Autodesk Inventor part; units mm, degrees
ref_plane "YZ Plane" through (0, 0, 0) normal (1, 0, 0) x (0, 1, 0)
ref_plane "XZ Plane" through (0, 0, 0) normal (0, 1, 0) x (-1, 0, 0)
ref_plane "XY Plane" through (0, 0, 0) normal (0, 0, 1) x (1, 0, 0)
sketch "Sketch1" plane through (0, 0, 0) normal (0, 0, 1) x (1, 0, 0)
  arc A0 (187.325, 0) -> (0, 187.325) centre (0, 0) ccw
  arc A1 (136.525, 0) -> (0, 136.525) centre (0, 0) ccw
  line L0 (0, 136.525) -> (0, 187.325)
  line L1 (136.525, 0) -> (187.325, 0)
  point P0 (161.925, 0)
  point P1 (0, 161.925)
  dimension "d2" = 187.325
  dimension "d3" = 136.525
extrude "Extrusion1" add sketch "Sketch1" along normal blind 0.4
sketch "Sketch3" plane through (0, 0, 0.4) normal (0, 0, 1) x (1, 0, 0)
  arc A0 (178.117, 32.1925) -> (181.231, 32.8119) centre (179.674, 32.5022) ccw
  line L0 (179.9922, 39.0399) -> (181.231, 32.8119)
  arc A1 (179.9922, 39.0399) -> (176.8782, 38.4205) centre (178.4352, 38.7302) ccw
  line L1 (178.117, 32.1925) -> (176.8782, 38.4205)
  line L2 (161.1024, 82.5109) -> (158.109, 88.1111)
  arc A2 (161.1024, 82.5109) -> (163.9025, 84.0076) centre (162.5024, 83.2593) ccw
  line L3 (160.9091, 89.6078) -> (163.9025, 84.0076)
  arc A3 (160.9091, 89.6078) -> (158.109, 88.1111) centre (159.5091, 88.8595) ccw
  circle A4 centre (156.6217, 0.5713) radius 5.334
  line L4 (84.0076, 163.9025) -> (89.6078, 160.9091)
  arc A5 (88.1111, 158.109) -> (89.6078, 160.9091) centre (88.8595, 159.5091) ccw
  line L5 (88.1111, 158.109) -> (82.5109, 161.1024)
  arc A6 (84.0076, 163.9025) -> (82.5109, 161.1024) centre (83.2593, 162.5024) ccw
  line L6 (32.8119, 181.231) -> (39.0399, 179.9922)
  arc A7 (38.4205, 176.8782) -> (39.0399, 179.9922) centre (38.7302, 178.4352) ccw
  line L7 (38.4205, 176.8782) -> (32.1925, 178.117)
  arc A8 (32.8119, 181.231) -> (32.1925, 178.117) centre (32.5022, 179.674) ccw
  circle A9 centre (88.0554, 129.5258) radius 5.334
  circle A10 centre (167.6741, 61.0284) radius 8.89
  circle A11 centre (167.6741, 61.0284) radius 14.2875
  point P0 (0, 0)
  dimension "d10" = 28.575
extrude "Extrusion2" cut sketch "Sketch3" against normal through all contours L1 A1 L0 A0 | L2 A3 L3 A2 | A4 | L4 A5 L5 A6 | L6 A7 L7 A8 | A9 | A10 | A11
fillet "Fillet1" radius 3.175 2 edges at (171.7808, 74.7129, 0.2) (179.6163, 53.1851, 0.2)
properties part number "3DPRINT,CABLE,TRAY" material "ABS Plastic"
Input: part model. Units: mm. Frame: model coordinates. Give positions to 0.01 mm unless a question says otherwise; leave off trailing zeros. Order: outer loops, then holes, each group sorted by start corner. A loop starts at its lowest first (then second) coordinate and runs counter-clockwise, first axis right, second up.
1. Line query: probe 1 along Y at (x, z) = (162.5, 0.25); probe 2 along Y at (x, z) = (36.5, 0.1); probe 3 along X at (y, z) = (159, 0.35). Output: solid intervals per line, ascending.
Computed:
probe 1: y = 0 to 47.71, 74.35 to 81.67, 86.63 to 93.19
probe 2: y = 131.56 to 177.26, 180.5 to 183.73
probe 3: x = 0 to 86.44, 90.36 to 99.04
2. Pin query (flat end, axial travel): pin 1 Ø8.5 at (x, y) = (156.62, 0.57) entering from -Z. Return the tip coordinate at first contact, or that it passes through.
Computed:
pin 1: passes through
3. Draft query along X for faces 1 (the face through (95.47, 97.593, 0.197)), 2 (the face through (100, 108, 0.4)), 3 (the face through (86.9, 124.32, 0.2)), 4 (the face through (99.09, 158.97, 0.2)). Return one class per face: released by +X, released by -X, zero draft, split by the parting line, or undercut.
Computed:
face 1: released by -X
face 2: zero draft
face 3: undercut
face 4: released by +X
4. Cut plane B-B (x = 54). Return loops of the section in (y, z).
Computed:
outline: (125.39, 0) - (179.37, 0) - (179.37, 0.4) - (125.39, 0.4) - close
5. Cut plane A-A (z = 0.1). State how many separate pieces and enclosed holes the cut face has, and give its area (3 significant figures).
Computed:
separate pieces: 1
enclosed holes: 5
area: 12,100 mm2
6. Cut plane C-C (y = 166.5). Return loops of the section in (x, z), and give its area (3 significant figures).
Computed:
outline: (0, 0) - (85.84, 0) - (85.84, 0.4) - (0, 0.4) - close
area: 34.3 mm2
